Autodesk Inventor part; units mm, degrees
ref_plane "YZ Plane" through (0, 0, 0) normal (1, 0, 0) x (0, 1, 0)
ref_plane "XZ Plane" through (0, 0, 0) normal (0, 1, 0) x (-1, 0, 0)
ref_plane "XY Plane" through (0, 0, 0) normal (0, 0, 1) x (1, 0, 0)
sketch "Náčrt1" plane through (0, 0, 0) normal (0, 0, 1) x (1, 0, 0)
  line L0 (0, 0) -> (33.3333, 0)
  line L1 (0, 19.335) -> (25, 19.335)
  line L2 (25, 19.335) -> (25, 16.5)
  line L3 (25, 16.5) -> (0, 16.5)
  line L4 (0, 16.5) -> (0, 19.335)
  dimension "d0" = 25
  dimension "d6" = 38.67
  dimension "d7" = 33
revolve "Rotace1" add sketch "Náčrt1" angle 360 about axis through (0, 0, 0) along (1, 0, 0)
chamfer "Zkosení1" distance 1 angle 45 2 edges at (25, -16.5, 0) (0, -16.5, 0)
chamfer "Zkosení2" distance 0.2 angle 45 1 edges at (0, -19.335, 0)
chamfer "Zkosení4" distance 2 angle 20 1 edges at (25, -19.335, 0) measured on face at (16.7333, 19.2723, -1.5558)
equation "\"Rozmer_A\" = d6"
equation "\"Rozmer_B\" = 0"
equation "\"Rozmer_C\" = 0"
equation "\"Rozmer_D\" = d0"
properties part number "NA-45-h-Crown-157" material "19 573.4"
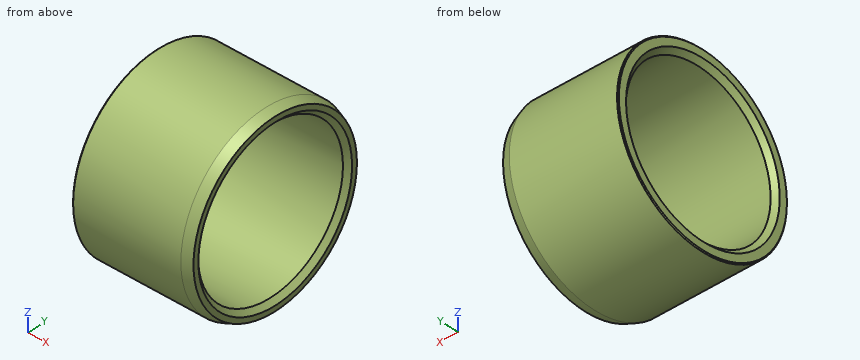
Design review of the part built by this model. Coordinates are the model's own, in mm. Give positions to 0.01 mm unless a question says otherwise; leave off trailing zeros. Order: outer loops, then holes, each group sorted by start corner. A loop starts at its lowest first (then second) coordinate and runs counter-clockwise, first axis right, second up.
1. Add section A-A, the plane y = 0. State the section outline as (x, z) points (3 decimals), then the cut area to 3 significant figures.
Solution:
outline: (0, -19.135) - (0.2, -19.335) - (23, -19.335) - (25, -18.607) - (25, -17.5) - (24, -16.5) - (1, -16.5) - (0, -17.5) - close; (0, 17.5) - (1, 16.5) - (24, 16.5) - (25, 17.5) - (25, 18.607) - (23, 19.335) - (0.2, 19.335) - (0, 19.135) - close
area: 138 mm2
2. To check wall thickness, follow L1, parallel to Z at x = 17.5, y = 0 (3 decimals); L2, parallel to Z at x = 10, y = -4.5; L3, parallel to Y at x = 14.5, z = -7.5. State the ranges of each line that lie inside material, in increasing order.
Solution:
L1: z = -19.335 to -16.5, 16.5 to 19.335
L2: z = -18.8 to -15.87, 15.87 to 18.8
L3: y = -17.82 to -14.7, 14.7 to 17.82
3. For pin 1 Ø5 at (x, y) = (18, -5.5) entering from +Z; pin 2 Ø8 at (x, z) = (4, -12.5) entering from -Y; pin 3 Ø12 at (x, y) = (2.5, -7) entering from +Z; pin 4 Ø12 at (y, z) = (-7.5, 4) entering from +X, all flat-tipped, find the tip position at first contact; note any pin that passes through.
Solution:
pin 1: stops at z = 19.1
pin 2: stops at y = -17.37
pin 3: stops at z = 19.31
pin 4: passes through
4. Add section C-C, the plane x = 3. State the section outline as (y, z) points (3 decimals).
Solution:
outline: circle Ø38.67 at (0, 0); hole circle Ø33 at (0, 0)
